Drawing for the job (mm, zero at the part's lowest x, y, z). A direction names the side the tool comes from. Give positions to 0.01 mm unless a question says otherwise; leave off trailing zeros. Loops run counter-clockwise (first coordinate to the right, second up) from the corner with the lowest first, then second, coordinate; pieces in that order, holes last. Notation, with made-up numbers: (3, 48.5) - (26, 48.5) arc R29 cw to (26, 68.5) - close; hole circle Ø9 at (86, 7). An arc over 180 degrees is marked (long way). Return JSON: item names as keys, results as strings. Group by question number.
1) Mould opens along Y. For the marked faces 1, 2 and 3 say: released by +Y, released by -Y, zero draft, split by the parting line, or undercut.
2) Slice it at A-A (y = 35). List the corners of the cut face in (x, z).
3) Drop flat-ended pins along their axis: pin 1 (1.5 mm diameter, centred on x = 3, y = 27.5, fed in from -Z); pin 2 (4 mm diameter, centred on x = 2, z = 22, fed in from +Y); pin 3 (3 mm diameter, centred on y = 9, z = 13, fed in from -X). Give the stop position or say it passes through.
4) Drill centre lines: probe 1 along Z at (x, y) = (7.75, 35); probe 2 along X at (y, z) = (56.5, 16); probe 3 along Y at (x, z) = (0.5, 8.5). Where is each one in solid material? Low to high. Write a range as from..to.
5) Slice it at C-C (x = 9.25). List the corners of the cut face in (y, z), and give its area (3 significant figures).
6) 3-axis set-ups, long thin cutter, end or side, ignore diameter. For the marked faces 4 and 5: which of +Z, -Z, +X, -X, +Y, -Y reach the whole face in a straight line?
7) Slice it at B-B (z = 16.5). List the corners of the cut face in (x, y).
8) Slice it at D-D (y = 57.5). List the corners of the cut face in (x, z).
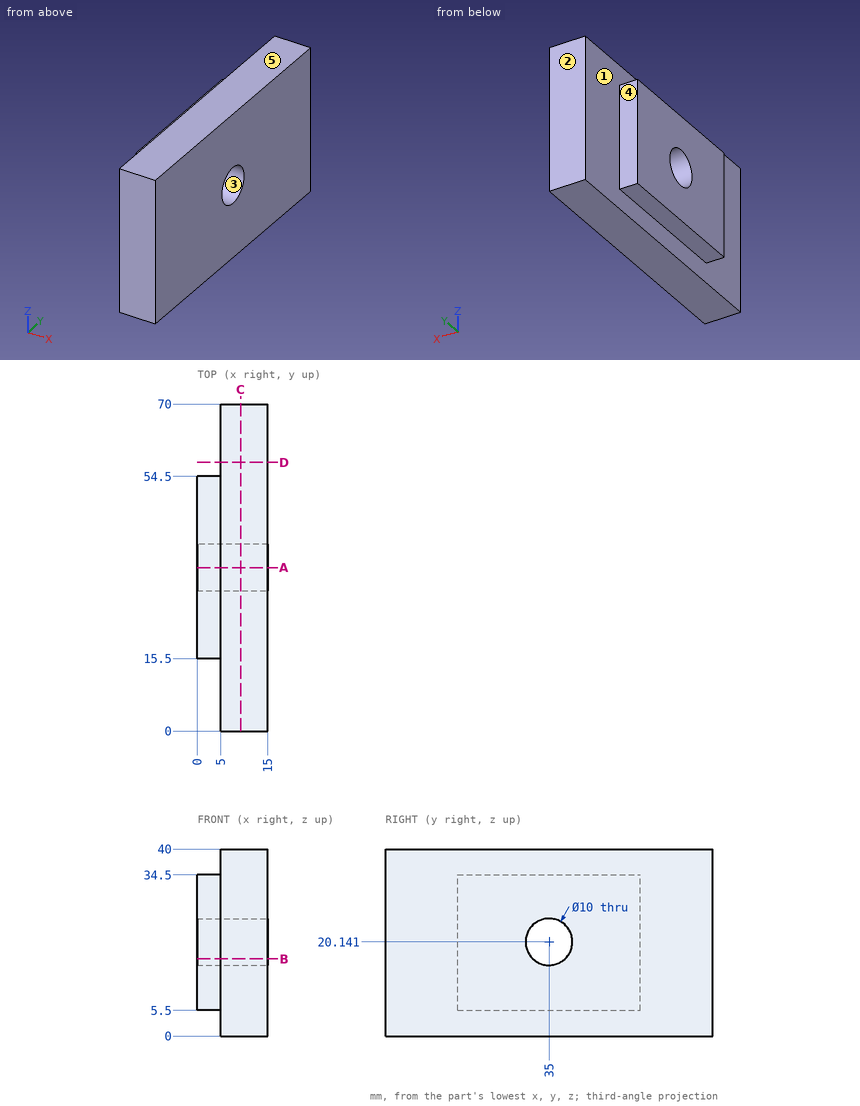
Results:
{
 "1": {"face 1": "zero draft", "face 2": "released by +Y", "face 3": "undercut"},
 "2": {"outline": "(0, 5.5) - (5, 5.5) - (5, 0) - (15, 0) - (15, 15.14) - (0, 15.14) - close; (0, 25.14) - (15, 25.14) - (15, 40) - (5, 40) - (5, 34.5) - (0, 34.5) - close"},
 "3": {"pin 1": "z = 5.5", "pin 2": "y = 54.5", "pin 3": "x = 5"},
 "4": {"probe 1": "0..15.14, 25.14..40", "probe 2": "5..15", "probe 3": "15.5..54.5"},
 "5": {"outline": "(0, 0) - (70, 0) - (70, 40) - (0, 40) - close; hole circle Ø10 at (35, 20.14)", "area": "2,720 mm2"},
 "6": {"face 4": "+Z, -Z, -X, +Y", "face 5": "+Z, +X, -X, +Y, -Y"},
 "7": {"outline": "(0, 15.5) - (5, 15.5) - (5, 0) - (15, 0) - (15, 31.57) - (0, 31.57) - close; (0, 38.43) - (15, 38.43) - (15, 70) - (5, 70) - (5, 54.5) - (0, 54.5) - close"},
 "8": {"outline": "(5, 0) - (15, 0) - (15, 40) - (5, 40) - close"}
}
